Solid Edge part; units mm, degrees
sketch "Sketch1" plane through (0, 0, 0) normal (0, -1, 0) x (1, 0, 0)
  line L0 (-13.7849, 36.6696) -> (-64.0155, 17.7868)
  arc A0 (-64.0155, 17.7868) -> (-72.1937, 18.2991) centre (-67.5343, 27.1472) cw
  line L1 (-93.2174, 29.3701) -> (-72.1937, 18.2991)
  arc A1 (-96.5723, 3.887) -> (-93.2174, 29.3701) centre (-99.6008, 17.2481) cw
  line L2 (-96.5723, 3.887) -> (-73.3996, 9.1394)
  arc A2 (-73.3996, 9.1394) -> (-64.3442, 6.677) centre (-71.1891, -0.6132) cw
  line L3 (-26.8148, -28.5596) -> (-64.3442, 6.677)
  arc A3 (-13.7849, 36.6696) -> (-26.8148, -28.5596) centre (0, 0) cw
  line L4 (-12.8348, 34.1423) -> (-63.0655, 15.2595)
  arc A4 (-63.0655, 15.2595) -> (-73.4518, 15.9101) centre (-67.5343, 27.1472) cw
  line L5 (-73.4518, 15.9101) -> (-94.4754, 26.981)
  arc A5 (-94.4754, 26.981) -> (-97.1692, 6.5202) centre (-99.6008, 17.2481) ccw
  line L6 (-97.1692, 6.5202) -> (-73.9965, 11.7726)
  arc A6 (-73.9965, 11.7726) -> (-62.4961, 8.6454) centre (-71.1891, -0.6132) cw
  line L7 (-62.4961, 8.6454) -> (-24.9666, -26.5912)
  arc A7 (-24.9666, -26.5912) -> (-12.8348, 34.1423) centre (0, 0) ccw
extrude "Protrusion1" add sketch "Sketch1" against normal blind 10
properties part number "1976-1200-C05" material "Poliuretano"
CAD build for the part. Positions are in the model's coordinates, mm. A direction names the side the tool comes from. Round coordinates to 2 decimals unless told otherwise and drop trailing zeros. Write each loop counter-clockwise with the first axis right and the second up, starting at its lowest first coordinate (ties: lowest second). Pieces come first, ordered by that corner, then holes.
(1) Slice it at C-C, the plane z = 0. Write the cut outline in (x, y) (3 decimals).
(2) Mould opens along X. For faces 1 (the face through (-37.599, 4.93, 24.833)), 2 (the face through (-42.4, 0, 23.4)), 3 (the face through (38.17, 4.93, -8.81)) say: pulls with the +X half, pulls with the -X half, needs draft (parallel to the pull), parting line crosses it, or undercut.
(3) Slice it at A-A, the plane x = 0. Write the cut outline in (y, z) (3 decimals), and give its area (3 significant figures).
(4) Probe line 1 along Z through (x, y) = (0, 2.75) (3 decimals); line 2 along X through (y, z) = (3.75, 0) (3 decimals); line 3 along Z through (x, y) = (-61, 1.25). List the from-to ranges inside material, lowest first.
(5) 3-axis set-ups, long thin cutter, end or side, ignore diameter. For faces 4 (the face through (-43.99, 4.93, -8.73)), 5 (the face through (-42.4, 10, 23.4)), 6 (the face through (-85.148, 4.93, 6.476)), 7 (the face through (-38.55, 4.93, 27.36)): which of +Z, -Z, +X, -X, +Y, -Y reach the whole face in a straight line?
(6) Drop flat-ended pins along their axis: P1, Ø2, axis at x = -11.5, y = 6, coming from the -Z side; P2, Ø3, axis at x = -25, y = 1, coming from the -Z side; P3, Ø2, axis at x = -41.5, y = 7.5, coming from the +Z side; P4, Ø12, axis at x = -91, z = -5.5, coming from the -Y side. Give the stop position or say it passes through.
From the geometry:
1. outline: (-57.233, 0) - (-53.288, 0) - (-53.288, 10) - (-57.233, 10) - close; (36.475, 0) - (39.175, 0) - (39.175, 10) - (36.475, 10) - close
2. face 1: undercut
2. face 2: needs draft
2. face 3: parting line crosses it
3. outline: (0, -39.175) - (10, -39.175) - (10, -36.475) - (0, -36.475) - close; (0, 36.475) - (10, 36.475) - (10, 39.175) - (0, 39.175) - close
3. area: 54.0 mm2
4. line 1: z = -39.175 to -36.475, 36.475 to 39.175
4. line 2: x = -57.233 to -53.288, 36.475 to 39.175
4. line 3: z = 3.54 to 7.24, 16.04 to 18.92
5. face 4: +Y, -Y
5. face 5: +Z, -Z, +X, -X, +Y
5. face 6: -Z, +Y, -Y
5. face 7: +Z, +Y, -Y
6. P1: stops at z = -37.74
6. P2: stops at z = -31.34
6. P3: stops at z = 26.63
6. P4: passes through
